Could you check a few things on this model? Use its own coordinates, in mm. Round coordinates to 2 decimals unless told otherwise and drop trailing zeros. Write each loop counter-clockwise with the first axis right and the second up, starting at its lowest first coordinate (ties: lowest second). Pieces come first, ordered by that corner, then holes. Notation, with made-up numbers: (20, 57) -> (51, 57) arc R28 ccw to (51, 93) -> close; hole circle Ø11 at (28.5, 65). An arc over 180 degrees is marked (long way). Answer in a Markdown table with one row per item. Add a question column.
```python
from build123d import *

# Parameters (mm, degrees)
SKETCH1_R               = 8
SKETCH1_R_2             = 6.9
BOSS_EXTRUDE1_DEPTH     = 135
CUT_EXTRUDE1_DEPTH      = 136.473244591
CUT_EXTRUDE1_DEPTH_BACK = 136.473244591
SKETCH3_R               = 2.6
SKETCH3_R_2             = 4.75
SKETCH3_R_3             = 1.6


with BuildPart() as part:
    # Sketch1 → Boss-Extrude1 (new body)
    with BuildSketch(Plane.XY):
        Circle(SKETCH1_R)
        Circle(SKETCH1_R_2, mode=Mode.SUBTRACT)
    extrude(amount=BOSS_EXTRUDE1_DEPTH)

    # Sketch3 → Cut-Extrude1 (cut, two sides: drawn at the far end of the back side and taken through both)
    with BuildSketch(Plane(origin=(0, 0, 0), x_dir=(1, 0, 0), z_dir=(0, 1, 0)).offset(-CUT_EXTRUDE1_DEPTH_BACK)):
        with Locations(Location((0, -100, 0), (0, 0, 270))):
            Circle(SKETCH3_R)
        with Locations(Location((0, -15.906910881, 0), (0, 0, 270))):
            Circle(SKETCH3_R_2)
        with Locations(Location((0, -3.406910881, 0), (0, 0, 270))):
            Circle(SKETCH3_R_3)
        with Locations(Location((0, -28.406910881, 0), (0, 0, 270))):
            Circle(SKETCH3_R_3)
    extrude(amount=CUT_EXTRUDE1_DEPTH + CUT_EXTRUDE1_DEPTH_BACK, mode=Mode.SUBTRACT)


solid = part.part
```
(1) Suppose I cut it at C-C, the plane x = 0. State how many separate pieces and enclosed holes the cut face has, then the cut area to 3 significant figures.
(2) If we mould it in two halves opening along Z, with no side actions, what happens to faces 1 (the face through (-1, 7.2, 102.4)), 2 (the face through (-6, -4, 0)), 3 (the face through (-6, -4, 135))? For each: pulls with the +Z half, pulls with the -Z half, needs draft (parallel to the pull), parting line crosses it, or undercut.
(3) Suppose I cut it at A-A, the plane y = 3.5. Please give me the cut outline in (x, z), then the cut area to 3 significant figures.
(4) For P1, Ø5, axis at y = -3.5, z = 89.5, coming from the -X side; P2, Ø1.5, axis at y = -5, z = 83.5, coming from the -X side; P3, Ø1.5, axis at y = -3, z = 90, coming from the -X side, each with a flat end and sliding along its axis, tell me the tip position at first contact or that it passes through.
(5) Suppose I cut it at B-B, the plane z = 100. Please give me the cut outline in (x, y), then the cut area to 3 significant figures.
(6) I need wall thicknesses on L1, parallel to Z at x = 0, y = 7.75; L2, parallel to X at y = 0.5, z = 120.5; L3, parallel to Y at x = 2.5, z = 125.5. Which ranges of each line are inside material? Lowest first, please.
Response:
| question | item | result |
|---|---|---|
| 1 | separate pieces | 10 |
| 1 | enclosed holes | 0 |
| 1 | area | 251 mm² |
| 2 | face 1 | undercut |
| 2 | face 2 | pulls with the -Z half |
| 2 | face 3 | pulls with the +Z half |
| 3 | outline | (-7.19, 0) -> (-5.95, 0) -> (-5.95, 135) -> (-7.19, 135) -> close; (5.95, 0) -> (7.19, 0) -> (7.19, 135) -> (5.95, 135) -> close |
| 3 | area | 337 mm² |
| 4 | P1 | x = -7.94 |
| 4 | P2 | x = -6.78 |
| 4 | P3 | x = -7.68 |
| 5 | outline | (-2.6, -7.57) -> (-2.6, -6.39) arc R6.9 cw to (-2.6, 6.39) -> (-2.6, 7.57) arc R8 ccw to start; (2.6, -7.57) arc R8 ccw to (2.6, 7.57) -> (2.6, 6.39) arc R6.9 cw to (2.6, -6.39) -> close |
| 5 | area | 39.8 mm² |
| 6 | L1 | 0 to 1.81, 5.01 to 11.16, 20.66 to 26.81, 30.01 to 97.4, 102.6 to 135 |
| 6 | L2 | -7.98 to -6.88, 6.88 to 7.98 |
| 6 | L3 | -7.6 to -6.43, 6.43 to 7.6 |
